Geometry check sheet. Reference: drawing and pictorial views, mm from the part's lowest x, y, z. A direction names the side the tool comes from. Round coordinates to 2 decimals unless told otherwise and drop trailing zeros. Write each loop counter-clockwise with the first axis right and the second up, starting at its lowest first coordinate (ties: lowest second). Pieces come first, ordered by that corner, then holes.
Item 1: Section check C-C, the plane z = 6. Record the cut outline in (x, y) (1 decimal).
Item 2: Release check for a two-part mould opening along X. For the marked faces 1, 2, 3 and 4 record: pulls with the +X half, pulls with the -X half, needs draft (parallel to the pull), parting line crosses it, or undercut.
Item 3: Section check B-B, the plane x = 5. Record the cut outline in (y, z), plus the area to 3 significant figures.
Item 4: Section check A-A, the plane y = 7. Record the cut outline in (x, z), plus the area to 3 significant figures.
Item 5: Set-up check for the marked faces 5 and 6: record each of +Z, -Z, +X, -X, +Y, -Y from which the full face is reachable in a straight line by a thin tool's end or side.
Item 6: Material ranges on line 1 along X through (y, z) = (8.25, 5.75); line 2 along Y through (x, z) = (8, 1); line 3 along Z through (x, y) = (5.75, 5.75) (1 decimal), recorded low to high.
Item 7: Depth check by flat-ended pin: pin 1 (3 mm diameter, centred on x = 5, y = 2, fed in from +Z); pin 2 (3 mm diameter, centred on x = 5, z = 4.33, fed in from -Y); pin 3 (3 mm diameter, centred on y = 4, z = 5.5, fed in from -X). Enter the tip coordinate at first touch or a pass-through.
Item 8: Section check D-D, the plane x = 8.5. Record the cut outline in (y, z).
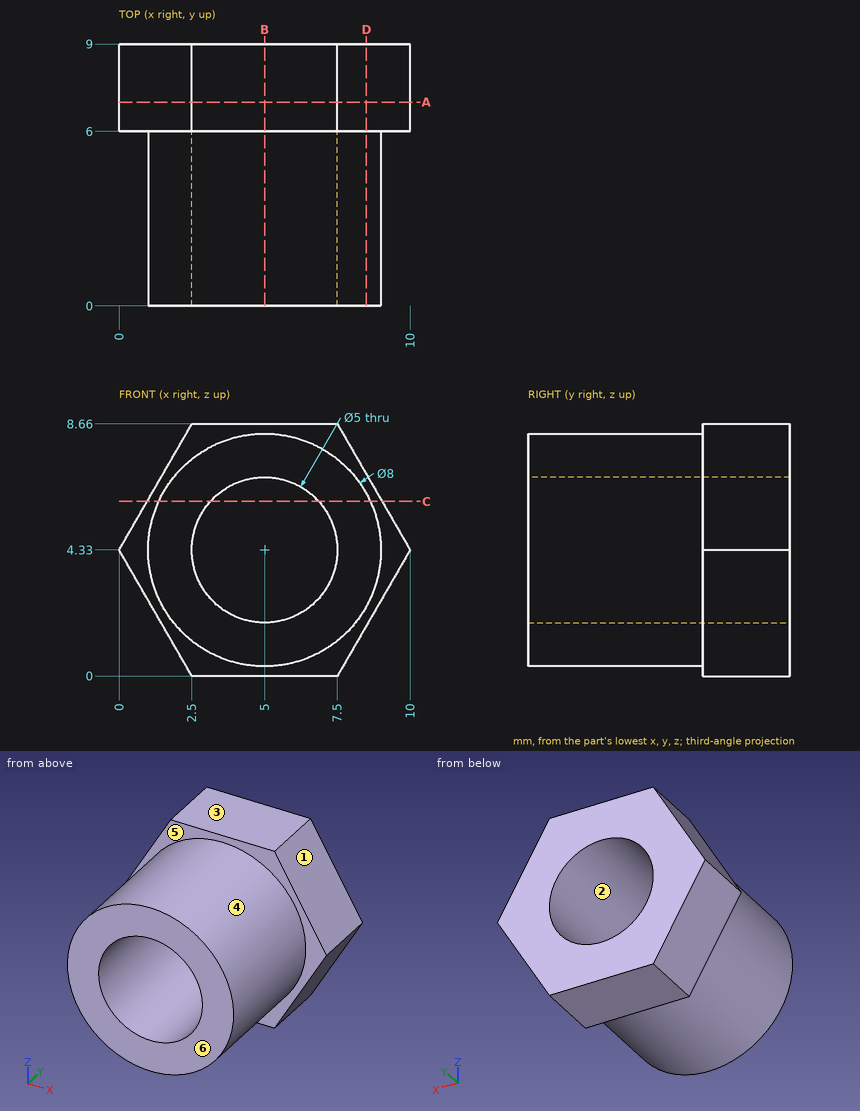
Values found:
1. outline: (1, 6) - (1.4, 6) - (1.4, 0) - (3.1, 0) - (3.1, 9) - (1, 9) - close; (6.9, 0) - (8.6, 0) - (8.6, 6) - (9, 6) - (9, 9) - (6.9, 9) - close
2. face 1: pulls with the +X half
2. face 2: undercut
2. face 3: needs draft
2. face 4: parting line crosses it
3. outline: (0, 0.33) - (6, 0.33) - (6, 0) - (9, 0) - (9, 1.83) - (0, 1.83) - close; (0, 6.83) - (9, 6.83) - (9, 8.66) - (6, 8.66) - (6, 8.33) - (0, 8.33) - close
3. area: 29.0 mm2
4. outline: (0, 4.33) - (2.5, 0) - (7.5, 0) - (10, 4.33) - (7.5, 8.66) - (2.5, 8.66) - close; hole circle Ø5 at (5, 4.33)
4. area: 45.3 mm2
5. face 5: -Y
5. face 6: +Z, -Z, +X, -X, -Y
6. line 1: x = 0.82 to 2.94, 7.06 to 9.18
6. line 2: y = 6 to 9
6. line 3: z = 0.4 to 1.9, 6.7 to 8.3
7. pin 1: stops at z = 8.33
7. pin 2: passes through
7. pin 3: stops at x = 1
8. outline: (0, 2.39) - (6, 2.39) - (6, 1.73) - (9, 1.73) - (9, 6.93) - (6, 6.93) - (6, 6.27) - (0, 6.27) - close
